```python
from build123d import *

# Parameters (mm, degrees)
F0_R      = 5.08
F1_DEPTH  = 190.5
F7_R      = 35.56
F8_DEPTH  = 10.16
F9_R      = 5.07999
F11_R     = 7.62
F12_DEPTH = 5.08
F13_R     = 2.53999
F14_R     = 5.08
F16_R     = 3.81


# Not quite as in the source:
# - a fillet or chamfer is up to 0.001 mm smaller than in the source, because OpenCascade refuses the exact size


with BuildPart() as f1:
    # F0 (on Top) → F1 (new body)
    with BuildSketch(Plane.XY):
        Circle(F0_R)
    extrude(amount=F1_DEPTH)

    # F7 (on offset) → F8 (join)
    with BuildSketch(Plane.XY.offset(129.54)):
        Circle(F7_R)
    extrude(amount=F8_DEPTH)

    # F9 (radius 5.08 in the source; OpenCascade refuses exactly that, so slightly less here)
    f9_edges = [f1.edges().sort_by_distance(p)[0] for p in [
        (-35.56, 0, 139.7),
        (-35.56, 0, 129.54),
    ]]
    fillet(f9_edges, radius=F9_R)

    # F14
    f14_edges = [f1.edges().sort_by_distance(p)[0] for p in [
        (-5.08, 0, 190.5),
    ]]
    fillet(f14_edges, radius=F14_R)

    # F16
    f16_edges = [f1.edges().sort_by_distance(p)[0] for p in [
        (-5.08, 0, 0),
    ]]
    fillet(f16_edges, radius=F16_R)


with BuildPart() as f12:
    # F11 (on offset) → F12 (new body)
    with BuildSketch(Plane.XY.offset(193.04)):
        Circle(F11_R)
    extrude(amount=F12_DEPTH)

    # F13 (radius 2.54 in the source; OpenCascade refuses exactly that, so slightly less here)
    f13_edges = [f12.edges().sort_by_distance(p)[0] for p in [
        (-7.62, 0, 193.04),
        (-7.62, 0, 198.12),
    ]]
    fillet(f13_edges, radius=F13_R)


solid = f1.part
```
Verification items for the finished model (mm, model axes). Coordinates: 2 decimals unless noted, no trailing zeros. Loops run counter-clockwise (first coordinate to the right, second up) from the corner with the lowest first, then second, coordinate; pieces in that order, holes last. Notation, with made-up numbers: (83, 74) -> (100, 74) arc R25 cw to (100, 108) -> close; hole circle Ø7 at (-12, 29.25). An arc over 180 degrees is marked (long way). Answer in a Markdown table with one row per item. Add a question column.
1. Draft check along X on faces 1 (the face through (6, 0, 129.54)), 2 (the face through (-0.661, 5.037, 65.795)). Enter one of: +X half, -X half, draft (parallel to the pull), parting line (faces both ways), or undercut.
2. Section check A-A, the plane z = 159. Enter the section's corners in (x, y), then the cut area to 3 significant figures.
3. Depth check by flat-ended pin: P1, Ø12, axis at y = 13, z = 108.5, coming from the -X side; P2, Ø8, axis at x = 2, y = -11.5, coming from the -Z side; P3, Ø10, axis at x = -2, y = 13.5, coming from the +Z side; P4, Ø12, axis at y = 6.5, z = 157.5, coming from the +X side. Enter the tip coordinate at first touch or a pass-through.
4. Material ranges on probe 1 along Z at (x, y) = (2.5, -6); probe 2 along Y at (x, z) = (0, 164.5); probe 3 along Z at (x, y) = (28.5, 14), recorded low to high. Write a range as [from, to].
Derived:
| question | item | result |
|---|---|---|
| 1 | face 1 | draft |
| 1 | face 2 | parting line |
| 2 | outline | circle Ø10.16 at (0, 0) |
| 2 | area | 81.1 mm² |
| 3 | P1 | passes through |
| 3 | P2 | stops at z = 129.54 |
| 3 | P3 | stops at z = 139.7 |
| 3 | P4 | stops at x = 5.06 |
| 4 | probe 1 | z = [129.54, 139.7] |
| 4 | probe 2 | y = [-5.08, 5.08] |
| 4 | probe 3 | z = [129.7, 139.54] |
